Geometry: final body of the model. Coordinates: model frame, mm. Face numbers are marked on the shaded views. A direction names the side the tool comes from. Give positions to 0.01 mm unless a question says otherwise; leave off trailing zeros. Loops run counter-clockwise (first coordinate to the right, second up) from the corner with the lowest first, then second, coordinate; pieces in that order, holes last. Notation, with made-up numbers: (-35.5, 31.25) - (15.5, 31.25) arc R34 ccw to (15.5, 67.25) - close; hole circle Ø7 at (-10.5, 43.5). An arc over 180 degrees is marked (long way). Use one line per item in the form item = value.
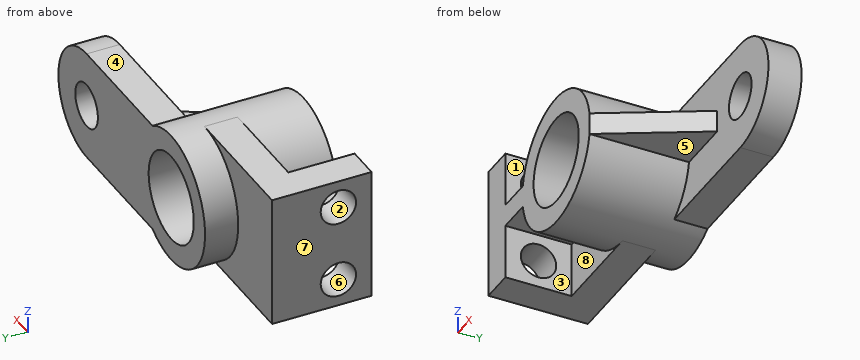
```python
from build123d import *

# Parameters (mm, degrees)
F0_W      = 60
F0_H      = 60
F1_DEPTH  = 45
F2_W      = 45
F2_H      = 25
F3_DEPTH  = 30
F4_R      = 8
F5_DEPTH  = 15
F6_R      = 8
F7_DEPTH  = 25
F8_R      = 30
F9_DEPTH  = 60
F10_R     = 20
F11_DEPTH = 60
F13_DEPTH = 15
F14_R     = 10
F15_DEPTH = 25
F17_DEPTH = 60
F19_DEPTH = 25


with BuildPart() as f1:
    # F0 (on Front) → F1 (new body)
    with BuildSketch(Plane.XZ):
        with Locations((-30, 30)):
            Rectangle(F0_W, F0_H)
    extrude(amount=F1_DEPTH)

    # F2 (on face) → F3 (cut)
    with BuildSketch(Plane.XZ.offset(45)):
        with Locations((-22.5, 12.5)):
            Rectangle(F2_W, F2_H)
        with Locations((-22.5, 47.5)):
            Rectangle(F2_W, F2_H)
    extrude(amount=-F3_DEPTH, mode=Mode.SUBTRACT)

    # F4 (on face) → F5 (cut)
    with BuildSketch(Plane.YZ.offset(-45)):
        with Locations((-30, 12.5)):
            Circle(F4_R)
    extrude(amount=-F5_DEPTH, mode=Mode.SUBTRACT)

    # F6 (on face) → F7 (cut)
    with BuildSketch(Plane.YZ.offset(-45)):
        with Locations((-30, 47.5)):
            Circle(F6_R)
    extrude(amount=-F7_DEPTH, mode=Mode.SUBTRACT)

    # F8 (on face) → F9 (join)
    with BuildSketch(Plane.XZ.offset(45)):
        with Locations((0, 30)):
            Circle(F8_R)
    extrude(amount=-F9_DEPTH)

    # F10 (on face) → F11 (cut)
    with BuildSketch(Plane.XZ.offset(45)):
        with Locations((0, 30)):
            Circle(F10_R)
    extrude(amount=-F11_DEPTH, mode=Mode.SUBTRACT)

    # F12 (on face) → F13 (join)
    with BuildSketch(Plane(origin=(0, 15, 0), x_dir=(-1, 0, 0), z_dir=(0, 1, 0))):
        with BuildLine():
            Line((-75, 5), (-75, 30))
            Line((-75, 30), (-75, 55))
            ThreePointArc((-75, 55), (-100, 30), (-75, 5))
        make_face()
        with BuildLine():
            Line((-75, 55), (-75, 30))
            Line((-75, 30), (-75, 5))
            Line((-75, 5), (-16.5831239518, 5))
            ThreePointArc((-16.5831239518, 5), (-30, 30), (-16.5831239518, 55))
            Line((-16.5831239518, 55), (-75, 55))
        make_face()
    extrude(amount=-F13_DEPTH)

    # F14 (on face) → F15 (cut)
    with BuildSketch(Plane.XZ):
        with Locations((75, 30)):
            Circle(F14_R)
    extrude(amount=-F15_DEPTH, mode=Mode.SUBTRACT)

    # F16 (on face) → F17 (join)
    with BuildSketch(Plane(origin=(0, 15, 0), x_dir=(-1, 0, 0), z_dir=(0, 1, 0))):
        with BuildLine():
            Line((-29.5803989155, 25), (-29.5803989155, 35))
            ThreePointArc((-29.5803989155, 35), (-30, 30), (-29.5803989155, 25))
        make_face()
        with BuildLine():
            ThreePointArc((-29.5803989155, 25), (-30, 30), (-29.5803989155, 35))
            Line((-29.5803989155, 35), (-54.5803989155, 35))
            Line((-54.5803989155, 35), (-54.5803989155, 25))
            Line((-54.5803989155, 25), (-29.5803989155, 25))
        make_face()
    extrude(amount=-F17_DEPTH)

    # F18 (on face) → F19 (cut)
    with BuildSketch(Plane(origin=(0, 0, 25), x_dir=(1, 0, 0), z_dir=(0, 0, -1))):
        Polygon((54.5803989155, 45), (29.5803989155, 45), (54.5803989155, 0), align=None)
    extrude(amount=-F19_DEPTH, mode=Mode.SUBTRACT)


solid = f1.part
```
(1) Pin query (flat end, axial travel): P1, Ø4.5, axis at x = -39.5, y = -36.5, coming from the -Z side; P2, Ø12, axis at x = 14, z = 41.5, coming from the +Y side; P3, Ø1, axis at x = -34, z = 44, coming from the +Y side; P4, Ø14.5, axis at y = -30, z = 12.5, coming from the +X side. Return the tip coordinate at first contact, or that it passes through.
Solution:
P1 = 25
P2 = 15
P3 = 0
P4 = 28.19
(2) Cut plane D-D (x = -12). Return the cut outline in (y, z), plus the area to 3 significant figures.
Solution:
outline = (-45, 2.5) - (-15, 2.5) - (-15, 0) - (0, 0) - (0, 2.5) - (15, 2.5) - (15, 14) - (-45, 14) - close; (-45, 46) - (15, 46) - (15, 57.5) - (0, 57.5) - (0, 60) - (-15, 60) - (-15, 57.5) - (-45, 57.5) - close
area = 1,450 mm2
(3) Access query for the marked faces 1, 2, 3, 4 and 5. Directions: +Z, -Z, +X, -X, +Y, -Y. A direction counts if a zero-diameter tool reaches every point of the face in a straight line with its end or side. Return the directions, or none.
Solution:
face_1 = +Z, -Y
face_2 = -X
face_3 = -Z, -Y
face_4 = +Z, +X, +Y, -Y
face_5 = -Z, +X, -Y
(4) Pull-direction query (X, two-part tool) for the marked faces 6, 7 and 8; classes: released by +X, released by -X, zero draft, split by the parting line, or undercut.
Solution:
face_6 = zero draft
face_7 = released by -X
face_8 = undercut
(5) Cut plane C-C (y = -5). Return the cut outline in (x, z), plus the area to 3 significant figures.
Solution:
outline = (-60, 0) - (0, 0) arc R30 ccw to (29.58, 25) - (51.8, 25) - (51.8, 35) - (29.58, 35) arc R30 ccw to (0, 60) - (-60, 60) - close; hole circle Ø40 at (0, 30)
area = 3,980 mm2
(6) Material intervals for L1, parallel to Z at x = -48.5, y = -30; L2, parallel to X at y = -33.5, z = 22; L3, parallel to Z at x = 75, y = 9, sorted ascending. Write a range as from..to.
Solution:
L1 = 0..4.5, 20.5..39.5, 55.5..60
L2 = -60..-45, -28.91..-18.33, 18.33..28.91
L3 = 5..20, 40..55
(7) Cut plane A-A (y = -30). Return the cut outline in (x, z).
Solution:
outline = (-60, 0) - (-45, 0) - (-45, 4.5) - (-60, 4.5) - close; (-60, 20.5) - (-45, 20.5) - (-45, 25) - (-29.58, 25) arc R30 ccw to (29.58, 25) - (37.91, 25) - (37.91, 35) - (29.58, 35) arc R30 ccw to (-29.58, 35) - (-45, 35) - (-45, 39.5) - (-60, 39.5) - close; (-60, 55.5) - (-45, 55.5) - (-45, 60) - (-60, 60) - close; hole circle Ø40 at (0, 30)
(8) Cut plane B-B (z = 16.5). Return the cut outline in (x, y), plus the area to 3 significant figures.
Solution:
outline = (-60, -45) - (-45, -45) - (-45, -36.93) - (-60, -36.93) - close; (-60, -23.07) - (-45, -23.07) - (-45, -15) - (-26.79, -15) - (-26.79, -45) - (-14.76, -45) - (-14.76, 15) - (-26.79, 15) - (-26.79, 0) - (-60, 0) - close; (14.76, -45) - (26.79, -45) - (26.79, 0) - (96.04, 0) - (96.04, 15) - (14.76, 15) - close
area = 3,220 mm2
